```python
from build123d import *

# Parameters (mm, degrees)
F1_DEPTH = 50
F2_DEPTH = 20
F5_DEPTH = 99.6315023101
F6_R     = 1.5
F7_DEPTH = 7.4226145035
F8_R     = 2.5
F9_DEPTH = 10.0478655756


with BuildPart() as f1:
    # F0 (on Right) → F1 (new body)
    with BuildSketch(Plane.YZ):
        with BuildLine():
            Line((10, -2.2239327878), (10, 2.2239327878))
            Line((10, 2.2239327878), (-10, 2.2239327878))
            Line((-10, 2.2239327878), (-10, -2.2239327878))
            Line((-10, -2.2239327878), (-2.6, -2.2239327878))
            Line((-2.6, -2.2239327878), (-2.6, -4.2239327878))
            Line((-2.6, -4.2239327878), (-5, -4.2239327878))
            Line((-5, -4.2239327878), (-5, -5.0419522724))
            ThreePointArc((-5, -5.0419522724), (-4.9238795325, -5.4246357048), (-4.7071067812, -5.7490590536))
            Line((-4.7071067812, -5.7490590536), (-2.9251262658, -7.531039569))
            ThreePointArc((-2.9251262658, -7.531039569), (-2.600702917, -7.7478123203), (-2.2180194847, -7.8239327878))
            Line((-2.2180194847, -7.8239327878), (2.2180194847, -7.8239327878))
            ThreePointArc((2.2180194847, -7.8239327878), (2.600702917, -7.7478123203), (2.9251262658, -7.531039569))
            Line((2.9251262658, -7.531039569), (4.7071067812, -5.7490590536))
            ThreePointArc((4.7071067812, -5.7490590536), (4.9238795325, -5.4246357048), (5, -5.0419522724))
            Line((5, -5.0419522724), (5, -4.2239327878))
            Line((5, -4.2239327878), (2.6, -4.2239327878))
            Line((2.6, -4.2239327878), (2.6, -2.2239327878))
            Line((2.6, -2.2239327878), (10, -2.2239327878))
        make_face()
    extrude(amount=-F1_DEPTH)

    # F0 (on Right) → F2 (join)
    with BuildSketch(Plane.YZ):
        with BuildLine():
            Line((10, -2.2239327878), (10, 2.2239327878))
            Line((10, 2.2239327878), (-10, 2.2239327878))
            Line((-10, 2.2239327878), (-10, -2.2239327878))
            Line((-10, -2.2239327878), (-2.6, -2.2239327878))
            Line((-2.6, -2.2239327878), (-2.6, -4.2239327878))
            Line((-2.6, -4.2239327878), (-5, -4.2239327878))
            Line((-5, -4.2239327878), (-5, -5.0419522724))
            ThreePointArc((-5, -5.0419522724), (-4.9238795325, -5.4246357048), (-4.7071067812, -5.7490590536))
            Line((-4.7071067812, -5.7490590536), (-2.9251262658, -7.531039569))
            ThreePointArc((-2.9251262658, -7.531039569), (-2.600702917, -7.7478123203), (-2.2180194847, -7.8239327878))
            Line((-2.2180194847, -7.8239327878), (2.2180194847, -7.8239327878))
            ThreePointArc((2.2180194847, -7.8239327878), (2.600702917, -7.7478123203), (2.9251262658, -7.531039569))
            Line((2.9251262658, -7.531039569), (4.7071067812, -5.7490590536))
            ThreePointArc((4.7071067812, -5.7490590536), (4.9238795325, -5.4246357048), (5, -5.0419522724))
            Line((5, -5.0419522724), (5, -4.2239327878))
            Line((5, -4.2239327878), (2.6, -4.2239327878))
            Line((2.6, -4.2239327878), (2.6, -2.2239327878))
            Line((2.6, -2.2239327878), (10, -2.2239327878))
        make_face()
        with BuildLine():
            Line((-10, 2.2239327878), (10, 2.2239327878))
            Line((10, 2.2239327878), (-83.8033707131, 185.1717589215))
            ThreePointArc((-83.8033707131, 185.1717589215), (-85.4691993199, 186.6301037549), (-87.6816926961, 186.5486933108))
            Line((-87.6816926961, 186.5486933108), (-87.8392769518, 186.4793179564))
            ThreePointArc((-87.8392769518, 186.4793179564), (-89.4267375498, 184.8203885461), (-89.376201468, 182.5248441568))
            Line((-89.376201468, 182.5248441568), (-10, 2.2239327878))
        make_face()
    extrude(amount=-F2_DEPTH)

    # F4 (on offset) → F5 (cut, through all)
    with BuildSketch(Plane.XZ.offset(-10)):
        Polygon((-20, 203.6575904285), (-20, 2), (-6, 202.6809155941), align=None)
    extrude(amount=F5_DEPTH, mode=Mode.SUBTRACT)

    # F6 (on face) → F7 (cut, through all)
    with BuildSketch(Plane.YZ):
        with Locations((-86.4729180545, 183.8029941528)):
            Circle(F6_R)
    extrude(amount=-F7_DEPTH, mode=Mode.SUBTRACT)

    # F8 (on face) → F9 (cut, through all)
    with BuildSketch(Plane.XY.offset(2.2239327878)):
        with Locations((-45, 0)):
            Circle(F8_R)
        with Locations((-30, 0)):
            Circle(F8_R)
    extrude(amount=-F9_DEPTH, mode=Mode.SUBTRACT)


solid = f1.part
```
Can you work these out from the model? Positions are in its coordinate system, mm. A direction names the side the tool comes from. Give positions to 0.01 mm unless a question says otherwise; leave off trailing zeros. Order: outer loops, then holes, each group sorted by start corner. A loop starts at its lowest first (then second) coordinate and runs counter-clockwise, first axis right, second up. Notation, with made-up numbers: M -2.75,-4.75 L 37.25,-4.75 A23 ccw 37.25,7.25 Z; hole C -2,-2 d6. An arc over 180 degrees is marked long. Write item = value, one per line. Start each with the question number.
Q1. Suppose I cut it at D-D (y = -45). Write out the boundary of the cut face in (x, z), plus the area to 3 significant figures.
Q2. I need wall thicknesses on probe 1 along X at (y, z) = (0, 0); probe 2 along Y at (x, z) = (-45, 0.25); probe 3 along Z at (x, y) = (-38, 3). Which ranges of each line are inside material? Lowest first, please. Write a range as [from, to].
Q3. Suppose I cut it at A-A (y = 0). Write out the boundary of the cut face in (x, z), plus the area to 3 significant figures.
Q4. For faces 1 (the flat face through (-25, -6, -2.224)), 2 (the flat face through (-48, 0, -7.824)), 3 (the flat face through (-25, -10, 0)), 4 (the flat face through (-25, 10, 0)), 5 (the flat face through (-35, 0, 2.224)), which set-ups out of +Z, -Z, +X, -X, +Y, -Y let a thin tool reach every point of the face, with its end or its side?
Q5. We'd pull the mould along X, two halves only. Please class faces 6 (the flat face through (-50, 0, -2)), 7 (the cylindrical face through (-32.5, 0.1, -2.7)), 8 (the flat face through (-25, 6, -2.224)): pulls with the +X half, pulls with the -X half, needs draft (parallel to the pull), parting line crosses it, or undercut.
Q6. Will these pins go through, and if not, where does the flat tip stop? pin 1 Ø8 at (x, y) = (-28.5, -7.5) entering from -Z; pin 2 Ø5 at (y, z) = (-33, 54.5) entering from +X; pin 3 Ø1 at (x, z) = (-35, -3.5) entering from -Y; pin 4 Ø3.5 at (y, z) = (-86.47, 183.8) entering from -X.
Q7. Suppose I cut it at B-B (x = -25). Write out the boundary of the cut face in (y, z), plus the area to 3 significant figures.
Q8. Suppose I cut it at C-C (z = 116). Write out the boundary of the cut face in (x, y).
Check result:
q1.outline = M -14.44,81.73 L 0,81.73 L 0,109.49 L -12.5,109.49 Z
q1.area = 374 mm2
q2.probe_1 = [-50, -47.5], [-42.5, -32.5], [-27.5, 0]
q2.probe_2 = [-10, -2.5], [2.5, 10]
q2.probe_3 = [-7.46, -4.22], [-2.22, 2.22]
q3.outline = M -50,-7.82 L -47.5,-7.82 L -47.5,2.22 L -50,2.22 Z; M -42.5,-7.82 L -32.5,-7.82 L -32.5,2.22 L -42.5,2.22 Z; M -27.5,-7.82 L 0,-7.82 L 0,21.73 L -18.62,21.73 L -20,2 L -20,2.22 L -27.5,2.22 Z
q3.area = 778 mm2
q4.face_1 = +X, -X, -Y
q4.face_2 = -Z, +X, -X, +Y, -Y
q4.face_3 = -Z, +X, -X, -Y
q4.face_4 = +Z, -Z, +X, -X, +Y
q4.face_5 = +Z, -X, +Y, -Y
q5.face_6 = pulls with the -X half
q5.face_7 = undercut
q5.face_8 = needs draft
q6.pin_1 = -6.96
q6.pin_2 = 0
q6.pin_3 = -2.6
q6.pin_4 = -7.44
q7.outline = M -10,-2.22 L -2.6,-2.22 L -2.6,-4.22 L -5,-4.22 L -5,-5.04 A1 ccw -4.71,-5.75 L -2.93,-7.53 A1 ccw -2.22,-7.82 L 2.22,-7.82 A1 ccw 2.93,-7.53 L 4.71,-5.75 A1 ccw 5,-5.04 L 5,-4.22 L 2.6,-4.22 L 2.6,-2.22 L 10,-2.22 L 10,2.22 L -10,2.22 Z
q7.area = 130 mm2
q8.outline = M -12.05,-60.09 L 0,-60.09 L 0,-48.34 L -12.05,-48.34 Z
